Geometry check sheet. Reference: the model listing, model coordinates, mm. A direction names the side the tool comes from. Round coordinates to 2 decimals unless told otherwise and drop trailing zeros. Loops run counter-clockwise (first coordinate to the right, second up) from the corner with the lowest first, then second, coordinate; pieces in that order, holes last. Notation, with made-up numbers: M 46,80 L 89,80 A11 ccw 89,92 Z; hole C 20.5,58 d2. An arc over 180 degrees is marked long. Write item = value, one per line.
from build123d import *

# Parameters (mm, degrees)
SKETCH1_W           = 100
SKETCH1_H           = 247
SKETCH1_R           = 1.525
SKETCH1_R_2         = 3.975
SKETCH1_R_3         = 1.5
BOSS_EXTRUDE1_DEPTH = 7
SKETCH2_R           = 11.025
CUT_EXTRUDE1_DEPTH  = 3
SKETCH4_W           = 100
SKETCH4_H           = 80
CUT_EXTRUDE3_DEPTH  = 134.421325132


with BuildPart() as part:
    # Sketch1 → Boss-Extrude1 (new body)
    with BuildSketch(Plane.XY):
        Rectangle(SKETCH1_W, SKETCH1_H)
        with Locations((-42, -34.5)):
            Circle(SKETCH1_R, mode=Mode.SUBTRACT)
        with Locations((42, -34.5)):
            Circle(SKETCH1_R, mode=Mode.SUBTRACT)
        with Locations((-42, -115.5)):
            Circle(SKETCH1_R, mode=Mode.SUBTRACT)
        with Locations((42, -115.5)):
            Circle(SKETCH1_R, mode=Mode.SUBTRACT)
        with Locations((0, 18.5)):
            Circle(SKETCH1_R_2, mode=Mode.SUBTRACT)
        with Locations((42, 115.5)):
            Circle(SKETCH1_R, mode=Mode.SUBTRACT)
        with Locations((-42, 115.5)):
            Circle(SKETCH1_R, mode=Mode.SUBTRACT)
        with Locations((-23.5, -65)):
            Circle(SKETCH1_R_3, mode=Mode.SUBTRACT)
        with Locations((-23.5, -112)):
            Circle(SKETCH1_R_3, mode=Mode.SUBTRACT)
        with Locations((23.5, -112)):
            Circle(SKETCH1_R_3, mode=Mode.SUBTRACT)
        with Locations((23.5, -65)):
            Circle(SKETCH1_R_3, mode=Mode.SUBTRACT)
        with BuildLine():
            Line((-19.05, -80.5), (-19.05, -86.5))
            ThreePointArc((-19.05, -86.5), (0, -105.55), (19.05, -86.5))
            Line((19.05, -86.5), (19.05, -80.5))
            ThreePointArc((19.05, -80.5), (0, -61.45), (-19.05, -80.5))
        make_face(mode=Mode.SUBTRACT)
    extrude(amount=BOSS_EXTRUDE1_DEPTH)

    # Sketch2 → Cut-Extrude1 (cut)
    with BuildSketch(Plane.XY.offset(7)):
        with Locations((0, 18.5)):
            Circle(SKETCH2_R)
    extrude(amount=-CUT_EXTRUDE1_DEPTH, mode=Mode.SUBTRACT)

    # Sketch4 → Cut-Extrude3 (cut, through all)
    with BuildSketch(Plane.XY.offset(7)):
        with Locations((0, 83.5)):
            Rectangle(SKETCH4_W, SKETCH4_H)
    extrude(amount=-CUT_EXTRUDE3_DEPTH, mode=Mode.SUBTRACT)


solid = part.part
(1) Material ranges on line 1 along Y through (x, z) = (23.5, 4.75); line 2 along Y through (x, z) = (0, 6.2) (3 decimals); line 3 along X through (y, z) = (-115.5, 4) (3 decimals), recorded low to high. Write a range as from..to.
Result set:
line_1 = -123.5..-113.5, -110.5..-66.5, -63.5..43.5
line_2 = -123.5..-105.55, -61.45..7.475, 29.525..43.5
line_3 = -50..-43.525, -40.475..40.475, 43.525..50
(2) Depth check by flat-ended pin: pin 1 Ø2.5 at (x, y) = (42, -115.5) entering from -Z; pin 2 Ø4 at (x, y) = (42, -34.5) entering from -Z. Enter the tip coordinate at first touch or a pass-through.
Result set:
pin_1 = through
pin_2 = 0
(3) Sectioned sample at B-B on x = 0. Record the cut outline in (y, z) (3 decimals).
Result set:
outline = M -123.5,0 L -105.55,0 L -105.55,7 L -123.5,7 Z; M -61.45,0 L 14.525,0 L 14.525,4 L 7.475,4 L 7.475,7 L -61.45,7 Z; M 22.475,0 L 43.5,0 L 43.5,7 L 29.525,7 L 29.525,4 L 22.475,4 Z
(4) Tool access check on faces 5 (the flat face through (-1, -39, 0)), 6 (the flat face through (5, 19, 4)), 7 (the cylindrical face through (-0.419, -105.545, 3.451)). Record the directions out of +Z, -Z, +X, -X, +Y, -Y that give a thin tool (end or side, any length) a straight path to the whole face; none if there is none.
Result set:
face_5 = -Z, +X, -X, +Y, -Y
face_6 = +Z
face_7 = +Z, -Z
(5) Release check for a two-part mould opening along Y. For faces 1 (the flat face through (-50, -41, 3)), 2 (the flat face through (-1, 43.5, 4)), 3 (the flat face through (-1, -123.5, 3)), 4 (the cylindrical face through (0.419, -61.455, 3.451)) record: released by +Y, released by -Y, zero draft, split by the parting line, or undercut.
Result set:
face_1 = zero draft
face_2 = released by +Y
face_3 = released by -Y
face_4 = undercut
(6) Sectioned sample at A-A on y = 18.5. Record the cut outline in (x, z) (3 decimals), then the cut area to 3 significant figures.
Result set:
outline = M -50,0 L -3.975,0 L -3.975,4 L -11.025,4 L -11.025,7 L -50,7 Z; M 3.975,0 L 50,0 L 50,7 L 11.025,7 L 11.025,4 L 3.975,4 Z
area = 602 mm2
